Source: CAD feature listing. Evaluate the final solid. Frame: model axes, mm. Coordinates: 2 decimals unless noted, no trailing zeros. Order: outer loops, then holes, each group sorted by start corner. A loop starts at its lowest first (then second) coordinate and runs counter-clockwise, first axis right, second up. Notation, with made-up numbers: (14, 15) -> (65, 15) arc R27 cw to (65, 35) -> close; hole circle Ø5 at (14.25, 66.5). An arc over 180 degrees is marked (long way). Write each question's results on one line, items separated by ' | '. Start each with the question number.
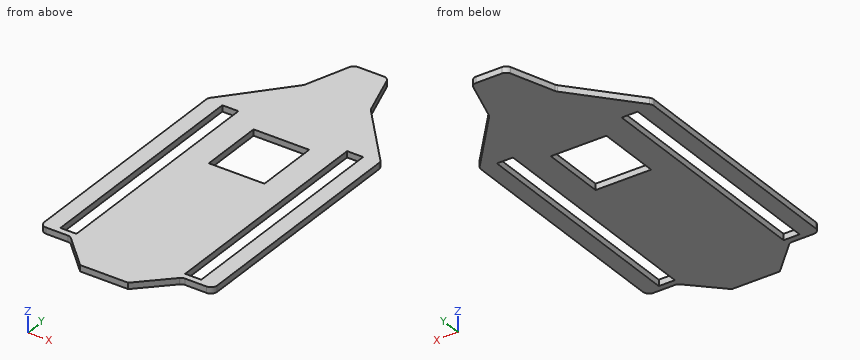
from build123d import *

# Parameters (mm, degrees)
SKETCH1_W           = 13
SKETCH1_H           = 188.148975749
BOSS_EXTRUDE1_DEPTH = 5
SKETCH2_W           = 45
SKETCH2_H           = 52
CUT_EXTRUDE1_DEPTH  = 341.122657523


with BuildPart() as part:
    # Sketch1 → Boss-Extrude1 (new body)
    with BuildSketch(Plane.XY):
        with BuildLine():
            Line((0, 30.859943174), (0, 219.008918923))
            ThreePointArc((0, 219.008918923), (0.311003468, 220.744808182), (1.205324608, 222.264750409))
            Line((1.205324608, 222.264750409), (42.261389271, 270.115641625))
            ThreePointArc((42.261389271, 270.115641625), (42.81710491, 270.906904614), (43.210130369, 271.790334282))
            Line((43.210130369, 271.790334282), (54.802396658, 306.567133147))
            ThreePointArc((54.802396658, 306.567133147), (56.605292439, 309.029920375), (59.503914938, 309.985818768))
            Line((59.503914938, 309.985818768), (80.378944352, 309.985818768))
            ThreePointArc((80.378944352, 309.985818768), (83.277566851, 309.029920375), (85.080462632, 306.567133147))
            Line((85.080462632, 306.567133147), (96.672728921, 271.790334282))
            ThreePointArc((96.672728921, 271.790334282), (97.06575438, 270.906904614), (97.621470019, 270.115641625))
            Line((97.621470019, 270.115641625), (138.677534682, 222.264750409))
            ThreePointArc((138.677534682, 222.264750409), (139.571855822, 220.744808182), (139.88285929, 219.008918923))
            Line((139.88285929, 219.008918923), (139.88285929, 30.859943174))
            ThreePointArc((139.88285929, 30.859943174), (138.418393196, 27.324409268), (134.88285929, 25.859943174))
            Line((134.88285929, 25.859943174), (117.446021446, 25.859943174))
            ThreePointArc((117.446021446, 25.859943174), (115.538843756, 25.481920377), (113.920048724, 24.405012478))
            Line((113.920048724, 24.405012478), (89.38285929, 0))
            Line((89.38285929, 0), (50.5, 0))
            Line((50.5, 0), (25.962810565, 24.405012478))
            ThreePointArc((25.962810565, 24.405012478), (24.344015534, 25.481920377), (22.436837844, 25.859943174))
            Line((22.436837844, 25.859943174), (5, 25.859943174))
            ThreePointArc((5, 25.859943174), (1.464466094, 27.324409268), (0, 30.859943174))
        make_face()
        with Locations((19.5, 124.934431049)):
            Rectangle(SKETCH1_W, SKETCH1_H, mode=Mode.SUBTRACT)
        with Locations((120.5, 124.934431049)):
            Rectangle(SKETCH1_W, SKETCH1_H, mode=Mode.SUBTRACT)
    extrude(amount=BOSS_EXTRUDE1_DEPTH)

    # Sketch2 → Cut-Extrude1 (cut, through all)
    with BuildSketch(Plane.XY.offset(5)):
        with Locations((69.88285929, 180.008918923)):
            Rectangle(SKETCH2_W, SKETCH2_H)
    extrude(amount=-CUT_EXTRUDE1_DEPTH, mode=Mode.SUBTRACT)


solid = part.part
(1) Section D-D on x = 75. Return the cut outline in (y, z), then the cut area to 3 significant figures.
(2) Line query: L1, parallel to X at y = 213, z = 0.35; L2, parallel to X at y = 204, z = 3.5; L3, parallel to Y at x = 66, z = 3.95. Output: solid intervals per line, ascending.
(3) First-contact query: P1, Ø1.5, axis at x = 121.5, z = 2, coming from the -Y side. Flat tip, straight axial feed; report the tip coordinate or a pass-through.
(4) Section B-B on z = 2.85. Count the separate pieces of the cut face and the enclosed holes in it, then the cut area to 3 significant figures.
(5) Section A-A on y = 180.5. Return the cut outline in (x, z), then the cut area to 3 significant figures.
(6) Section C-C on y = 70. Return the cut outline in (x, z).
Results list:
1) outline: (0, 0) -> (154.01, 0) -> (154.01, 5) -> (0, 5) -> close; (206.01, 0) -> (309.99, 0) -> (309.99, 5) -> (206.01, 5) -> close | area: 1,290 mm²
2) L1: x = 0 to 13, 26 to 114, 127 to 139.88 | L2: x = 0 to 13, 26 to 47.38, 92.38 to 114, 127 to 139.88 | L3: y = 0 to 154.01, 206.01 to 309.99
3) P1: stops at y = 25.86
4) separate pieces: 1 | enclosed holes: 3 | area: 28,200 mm²
5) outline: (0, 0) -> (13, 0) -> (13, 5) -> (0, 5) -> close; (26, 0) -> (47.38, 0) -> (47.38, 5) -> (26, 5) -> close; (92.38, 0) -> (114, 0) -> (114, 5) -> (92.38, 5) -> close; (127, 0) -> (139.88, 0) -> (139.88, 5) -> (127, 5) -> close | area: 344 mm²
6) outline: (0, 0) -> (13, 0) -> (13, 5) -> (0, 5) -> close; (26, 0) -> (114, 0) -> (114, 5) -> (26, 5) -> close; (127, 0) -> (139.88, 0) -> (139.88, 5) -> (127, 5) -> close
